```python
from build123d import *

# Parameters (mm, degrees)
F0_W     = 101.6
F0_H     = 50.8
F0_R     = 3.175
F1_DEPTH = 9.525
F2_SIZE2 = 1.27
F2_SIZE  = 1.27


with BuildPart() as f1:
    # F0 (on Top) → F1 (new body)
    with BuildSketch(Plane.XY):
        Rectangle(F0_W, F0_H)
        with Locations((-38.1, -19.05)):
            Circle(F0_R, mode=Mode.SUBTRACT)
        with Locations((38.1, -19.05)):
            Circle(F0_R, mode=Mode.SUBTRACT)
        with Locations((-38.1, 19.05)):
            Circle(F0_R, mode=Mode.SUBTRACT)
        with Locations((38.1, 19.05)):
            Circle(F0_R, mode=Mode.SUBTRACT)
    extrude(amount=-F1_DEPTH)

    # F2
    f2_edges = [f1.edges().sort_by_distance(p)[0] for p in [
        (-50.8, 0, 0),
        (0, -25.4, 0),
        (0, 25.4, 0),
        (50.8, 0, 0),
    ]]
    chamfer(f2_edges, length=F2_SIZE, length2=F2_SIZE2)


solid = f1.part
```
The listing builds one solid part. Answer for the finished solid, in the listing's coordinates (mm). Coordinates: 2 decimals unless noted, no trailing zeros. Loops run counter-clockwise (first coordinate to the right, second up) from the corner with the lowest first, then second, coordinate; pieces in that order, holes last. Notation, with made-up numbers: M 78,44.25 L 109,44.25 A14 ccw 109,61.25 Z; hole C 18.5,67.25 d11. An arc over 180 degrees is marked long. Answer as a JSON object with one key per item and string values. Group by question number.
Item 1: Section C-C (x = -38.1) is taken. Write down the section's boundary in (y, z) (3 decimals).
Item 2: Determine the mould class of faces 1 (the face through (-1, 25.4, -5)), 2 (the face through (-50.8, 0, -5)), 3 (the face through (-41.27, -18.91, -4.7)) for opening direction Y: +Y half, -Y half, draft (parallel to the pull), parting line (faces both ways), or undercut.
Item 3: This flat-tipped pin is pushed along its axis until it touches: P1, Ø5, axis at x = -38.1, y = -19.05, coming from the +Z side. Where does it stop, or does it pass through?
Item 4: Consider L1, parallel to Y at x = -38.1, z = -2.5 (3 decimals); L2, parallel to X at y = -19, z = -8.75; L3, parallel to X at y = -21.5, z = -3.5. Determine where each line is inside the solid, lowest interval first.
Item 5: Section A-A (z = -2.25) is taken. Write down the section's boundary in (x, y) (3 decimals), and give its area (3 significant figures).
Item 6: Section B-B (y = -19.05) is taken. Write down the section's boundary in (x, z) (3 decimals), and give its area (3 significant figures).
Solved:
{
 "1": {"outline": "M -25.4,-9.525 L -22.225,-9.525 L -22.225,0 L -24.13,0 L -25.4,-1.27 Z; M -15.875,-9.525 L 15.875,-9.525 L 15.875,0 L -15.875,0 Z; M 22.225,-9.525 L 25.4,-9.525 L 25.4,-1.27 L 24.13,0 L 22.225,0 Z"},
 "2": {"face 1": "+Y half", "face 2": "draft", "face 3": "undercut"},
 "3": {"P1": "passes through"},
 "4": {"L1": "y = -25.4 to -22.225, -15.875 to 15.875, 22.225 to 25.4", "L2": "x = -50.8 to -41.27, -34.93 to 34.93, 41.27 to 50.8", "L3": "x = -50.8 to -40.12, -36.08 to 36.08, 40.12 to 50.8"},
 "5": {"outline": "M -50.8,-25.4 L 50.8,-25.4 L 50.8,25.4 L -50.8,25.4 Z; hole C -38.1,-19.05 d6.35; hole C -38.1,19.05 d6.35; hole C 38.1,-19.05 d6.35; hole C 38.1,19.05 d6.35", "area": "5,030 mm2"},
 "6": {"outline": "M -50.8,-9.525 L -41.275,-9.525 L -41.275,0 L -49.53,0 L -50.8,-1.27 Z; M -34.925,-9.525 L 34.925,-9.525 L 34.925,0 L -34.925,0 Z; M 41.275,-9.525 L 50.8,-9.525 L 50.8,-1.27 L 49.53,0 L 41.275,0 Z", "area": "845 mm2"}
}
